Autodesk Inventor part; units mm, degrees
ref_plane "Work Plane1" through (0, 0, 0) normal (0, 0, 1) x (1, 0, 0)
ref_plane "YZ Plane" through (0, 0, 0) normal (1, 0, 0) x (0, 1, 0)
ref_plane "XZ Plane" through (0, 0, 0) normal (0, 1, 0) x (-1, 0, 0)
ref_plane "Work Plane1" through (0, 0, 0) normal (0, 0, 1) x (1, 0, 0)
sketch "Sketch1" plane through (0, 0, 0) normal (0, 0, 1) x (1, 0, 0)
  line L0 (-507.2437, -32.9396) -> (89.7639, -92.7893) construction
  arc A0 (22.3112, -84.0063) -> (-126.1247, 408.4057) centre (-651.3316, -18.4949) ccw construction
  line L1 (-74.7461, 453.0192) -> (-539.2143, 73.1912) construction
  line L2 (46.1596, 196.9837) -> (49.0458, 187.4093) construction
  arc A1 (75.0276, -91.312) -> (47.6027, 192.1965) centre (-651.3316, -18.4949) ccw
  arc A2 (47.6027, 192.1965) -> (-86.2286, 443.6292) centre (-651.3316, -18.4949) ccw
  arc A3 (22.1136, -86.0074) -> (-127.3954, 409.9642) centre (-651.3316, -18.4949) ccw
  line L3 (75.0276, -91.312) -> (22.1136, -86.0074)
  line L4 (-86.2286, 443.6292) -> (-127.3954, 409.9642)
  point P0 (0, 0)
extrude "Extrusion1" add sketch "Sketch1" along normal blind 4
properties part number "externalSupportRear1" material "Wood (Cherry)"
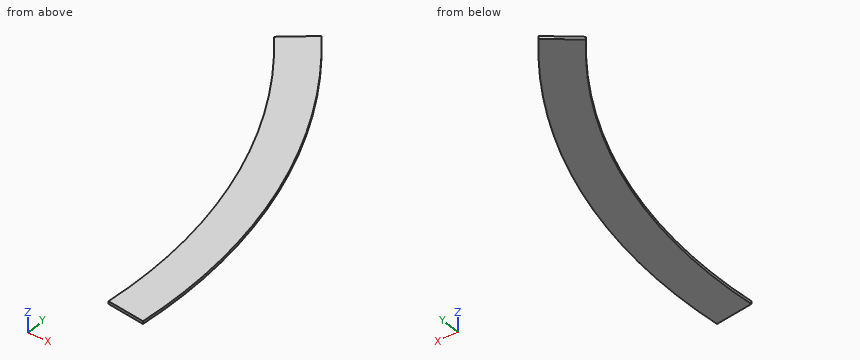
Model file for the job. Use its own axes, mm. Coordinates: 2 decimals unless noted, no trailing zeros. Order: outer loops, then holes, each group sorted by start corner. A loop starts at its lowest first (then second) coordinate and runs counter-clockwise, first axis right, second up. Notation, with made-up numbers: (87.5, -21.5) -> (97.5, -21.5) arc R29 cw to (97.5, 5.5) -> close; hole circle Ø7 at (7.5, 78). An arc over 180 degrees is marked (long way). Answer as a JSON object with one key per item and string values. Group by question number.
1) Drill centre lines: L1, parallel to X at y = -20.5, z = 1; L2, parallel to X at y = 130, z = 0.7; L3, parallel to Y at x = -98, z = 3.05. Where is each one in solid material? Low to high.
2) Cut at B-B, the plane y = 22.5. Write the cut outline in (x, z), then the cut area to 3 significant figures.
3) Cut at A-A, the plane z = 1.2. Write the cut outline in (x, y), then the cut area to 3 significant figures.
4) Flat gauge pin, fed straight in: pin 1 (1.5 mm diameter, centred on y = 114, z = 3, fed in from -X). Where does the tip first touch, or does it go through?
5) Cut at C-C, the plane x = -13. Write the cut outline in (y, z), then the cut area to 3 significant figures.
Check values:
{
 "1": {"L1": "x = 25.49 to 78.67", "L2": "x = 9 to 63.41", "L3": "y = 371.26 to 434"},
 "2": {"outline": "(24.25, 0) -> (77.52, 0) -> (77.52, 4) -> (24.25, 4) -> close", "area": "213 mm²"},
 "3": {"outline": "(-127.4, 409.96) arc R676.82 cw to (22.11, -86.01) -> (75.03, -91.31) arc R730 ccw to (47.6, 192.2) arc R730 ccw to (-86.23, 443.63) -> close", "area": "29,400 mm²"},
 "4": {"pin 1": "stops at x = 12.24"},
 "5": {"outline": "(206.49, 0) -> (335.67, 0) -> (335.67, 4) -> (206.49, 4) -> close", "area": "517 mm²"}
}
